Design review of the part built by this model. Coordinates are the model's own, in mm. Round coordinates to 2 decimals unless told otherwise and drop trailing zeros. Order: outer loops, then holes, each group sorted by start corner. A loop starts at its lowest first (then second) coordinate and runs counter-clockwise, first axis right, second up. Notation, with made-up numbers: M -30,9 L 5,9 A13 cw 5,29 Z; hole C 84,-28 d6. An arc over 180 degrees is marked long. Write each question's results on one line, items separated by ' | '. Start each with the question number.
Item 1: Take a section at A-A, the plane x = 0. Count the separate pieces of the cut face and the enclosed holes in it, plus the area to 3 significant figures.
Item 2: The part is to be moulded in two halves that separate along X. For faces 1 (the flat face through (0, -5, 0)), 2 (the flat face through (-12.7, 0, 5)), 3 (the cylindrical face through (5.005, 83.275, 4.696)), 4 (the cylindrical face through (0.14, -92.32, 4.7)), say which applies: +X half, -X half, draft (parallel to the pull), parting line (faces both ways), or undercut.
Item 3: Take a section at B-B, the plane y = -68. Write out the cut boundary in (x, z) (3 decimals).
Item 4: Wall thickness on line 1 (Y direction, x = 0, z = 5.5); line 2 (Y direction, x = -6.5, z = 2.5); line 3 (X direction, y = 81, z = 4.5): over which ranges is each line inside the solid? List them lowest first. Write a range as [from, to].
Item 5: Clearance check with a flat-ended pin moving along its axis: pin 1 (5 mm diameter, centred on x = 13.5, z = 8.5, fed in from +Y). State where the tip first meets the part, or that it passes through.
Solid Edge part; units mm, degrees
sketch "Sketch1" plane through (0, 0, 0) normal (0, 0, 1) x (1, 0, 0)
  line L0 (12.7, -88.9038) -> (12.7, 88.8962)
  line L1 (12.7, 88.8962) -> (-12.7, 88.8962)
  line L2 (-12.7, 88.8962) -> (-12.7, -88.9038)
  line L3 (-12.7, -88.9038) -> (-19.1158, -100.0163)
  line L4 (-19.1158, -100.0163) -> (-10.8669, -104.7788)
  line L5 (-10.8669, -104.7788) -> (0, -93.9119)
  line L6 (10.8669, -104.7788) -> (0, -93.9119)
  line L7 (19.1158, -100.0163) -> (10.8669, -104.7788)
  line L8 (12.7, -88.9038) -> (19.1158, -100.0163)
  dimension "D1" = 12.7
  dimension "D2" = 12.7
  dimension "D3" = 19.1158
extrude "Protrusion1" add sketch "Sketch1" along normal blind 9.525
hole "Hole_1" at (0, 76.1962, 0) direction (0, 0, 1) diameter 9.525 end up to next
fillet "Round_1" radius 3.175 2 edges at (12.7, 88.8962, 4.7625) (-12.7, 88.8962, 4.7625)
hole "Hole_2" at (-5.6127, 70.5835, 0) direction (0, 0, 1) diameter 3.175 end up to next
hole "Hole1" at (5.6127, 70.5835, 0) direction (0, 0, 1) diameter 3.175 end up to next
hole "Hole2" at (5.6127, 81.8088, 0) direction (0, 0, 1) diameter 3.175 end up to next
hole "Hole3" at (-5.6127, 81.8088, 0) direction (0, 0, 1) diameter 3.175 end up to next
fillet "Round_2" radius 12.7 2 edges at (10.8669, -104.7788, 4.7625) (-10.8669, -104.7788, 4.7625)
hole "Hole_6" at (0, -89.1494, 0) direction (0, 0, 1) diameter 6.35 end up to next
fillet "Round_3" radius 6.35 3 edges at (0, -93.9119, 4.7625) (12.7, -88.9038, 4.7625) (-12.7, -88.9038, 4.7625)
chamfer "Chamfer_1" distance 2.54 angle 45 2 edges at (-19.1158, -100.0163, 4.7625) (19.1158, -100.0163, 4.7625)
properties part number "SPaRC 02 - 004"
Results list:
1) separate pieces: 3 | enclosed holes: 0 | area: 1,610 mm²
2) face 1: draft | face 2: -X half | face 3: undercut | face 4: undercut
3) outline: M -12.7,0 L 12.7,0 L 12.7,9.525 L -12.7,9.525 Z
4) line 1: [-96.52, -92.32], [-85.97, 71.43], [80.96, 88.9] | line 2: [-99.84, 69.27], [71.9, 80.49], [83.13, 88.9] | line 3: [-12.7, -6.98], [-4.25, 4.25], [6.98, 12.7]
5) pin 1: y = 88.53
